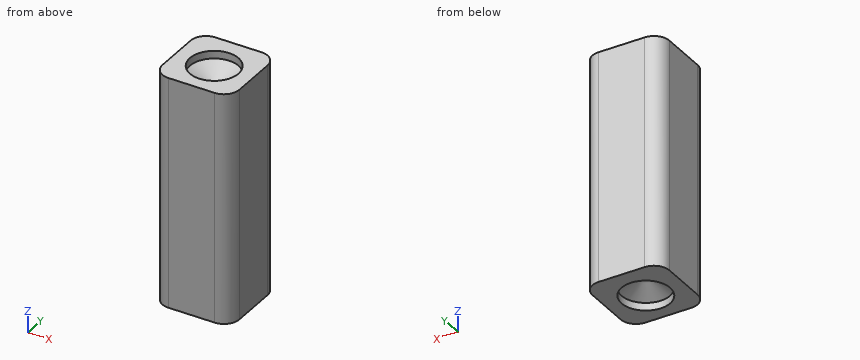
```python
from build123d import *

# Parameters (mm, degrees)
F0_W     = 25
F0_H     = 25
F1_DEPTH = 75
F4_D     = 15.8
F4_DEPTH = 2.5
F4_TIP   = 4.7467988903
F5_D     = 15.8
F5_DEPTH = 2.5
F5_TIP   = 4.7467988903
F6_R     = 5


with BuildPart() as f1:
    # F0 (on Top) → F1 (new body)
    with BuildSketch(Plane.XY):
        with Locations((0, 0.4354127725)):
            Rectangle(F0_W, F0_H)
    extrude(amount=F1_DEPTH)

    # F4
    with Locations(Plane(origin=(0, 0, 0), x_dir=(1, 0, 0), z_dir=(0, 0, -1))):
        with Locations((0, 0)):
            Hole(F4_D / 2, depth=F4_DEPTH)
            with Locations((0, 0, -(F4_DEPTH + F4_TIP / 2))):  # 118° drill point
                Cone(0, F4_D / 2, F4_TIP, mode=Mode.SUBTRACT)

    # F5
    with Locations(Plane.XY.offset(75)):
        with Locations((0, 0)):
            Hole(F5_D / 2, depth=F5_DEPTH)
            with Locations((0, 0, -(F5_DEPTH + F5_TIP / 2))):  # 118° drill point
                Cone(0, F5_D / 2, F5_TIP, mode=Mode.SUBTRACT)

    # F6
    f6_edges = [f1.edges().sort_by_distance(p)[0] for p in [
        (-12.5, 12.935413, 37.5),
        (-12.5, -12.064587, 37.5),
        (12.5, -12.064587, 37.5),
        (12.5, 12.935413, 37.5),
    ]]
    fillet(f6_edges, radius=F6_R)


solid = f1.part
```
The listing builds one solid part. Answer for the finished solid, in the listing's coordinates (mm). Give positions to 0.01 mm unless a question says otherwise; leave off trailing zeros. Order: outer loops, then holes, each group sorted by start corner. A loop starts at its lowest first (then second) coordinate and runs counter-clockwise, first axis right, second up. Notation, with made-up numbers: M 11.25,-17 L 38.25,-17 A17 ccw 38.25,-4 Z; hole C 66,-8.5 d10. An arc over 180 degrees is marked long. Put each result on its own line as item: value. Start each with the question number.
Item 1: The part is cut by section B-B, the plane x = 9.75. Determine the outline of the cut face in (y, z), and give its area (3 significant figures).
Item 2: The part is cut by section A-A, the plane z = 18. Determine the outline of the cut face in (x, y), and give its area (3 significant figures).
Item 3: Find the intervals of material crossed by line 1 along Y through (x, z) = (0, 74.4); line 2 along X through (y, z) = (0, 73.55); line 3 along X through (y, z) = (-7.5, 27.5), in increasing order.
Item 4: Flat-ended cylindrical pins translate along their axes: P1, Ø2, axis at y = 9, z = 60.5, coming from the -X side; P2, Ø4, axis at x = -4.5, y = 1, coming from the -Z side; P3, Ø1, axis at x = -8.5, z = 29, coming from the +Y side; P4, Ø1, axis at x = 5, y = 4, coming from the -Z side. Find the tip coordinate at first contact, or state that the pin passes through.
Item 5: The part is cut by section C-C, the plane y = -10. Determine the outline of the cut face in (x, z), and give its area (3 significant figures).
Answer key:
1. outline: M -11.53,0 L 12.4,0 L 12.4,75 L -11.53,75 Z
1. area: 1,790 mm²
2. outline: M -12.5,-7.06 A5 ccw -7.5,-12.06 L 7.5,-12.06 A5 ccw 12.5,-7.06 L 12.5,7.94 A5 ccw 7.5,12.94 L -7.5,12.94 A5 ccw -12.5,7.94 Z
2. area: 604 mm²
3. line 1: y = -12.06 to -7.9, 7.9 to 12.94
3. line 2: x = -12.5 to -7.9, 7.9 to 12.5
3. line 3: x = -12.48 to 12.48
4. P1: stops at x = -12.5
4. P2: stops at z = 3.28
4. P3: stops at y = 12.91
4. P4: stops at z = 3.1
5. outline: M -11.55,0 L 11.55,0 L 11.55,75 L -11.55,75 Z
5. area: 1,730 mm²
